from build123d import *

# Parameters (mm, degrees)
SKETCH2_R            = 13
SKETCH2_R_2          = 10
BOSS_EXTRUDE3_DEPTH  = 100
SKETCH2_3_R          = 14.5
SKETCH2_3_R_2        = 13
BOSS_EXTRUDE5_DEPTH  = 10
SKETCH8_R            = 25
BOSS_EXTRUDE7_DEPTH  = 6
SKETCH11_R           = 5.5
BOSS_EXTRUDE12_DEPTH = 10
SKETCH14_W           = 47.941155358
SKETCH14_H           = 10.12177459
CUT_EXTRUDE2_DEPTH   = 112.740771431
FILLET1_START        = -12.0000001
FILLET1_2_DEPTH      = 2.0000001
FILLET1_START_2      = 3.060887195
FILLET1_3_DEPTH      = 2.0000001
FILLET1_START_3      = -5.060887295
FILLET1_4_DEPTH      = 2
FILLET1_START_4      = 10
FILLET1_5_DEPTH      = 2
FILLET1_START_5      = -10
FILLET1_6_DEPTH      = 4.939112705
FILLET1_START_6      = 5.060887295
FILLET1_7_DEPTH      = 4.939112705
FILLET1_START_7      = -21.9089024
FILLET1_8_DEPTH      = 43.8178047


with BuildPart() as part:
    # Sketch2 → Boss-Extrude3 (new body)
    with BuildSketch(Plane(origin=(0, 0, 0), x_dir=(1, 0, 0), z_dir=(0, 1, 0))):
        with Locations(Location((0, 0, 0), (0, 0, 270))):
            Circle(SKETCH2_R)
        with Locations(Location((0, 0, 0), (0, 0, 270))):
            Circle(SKETCH2_R_2, mode=Mode.SUBTRACT)
    extrude(amount=BOSS_EXTRUDE3_DEPTH)

    # Sketch2<3> → Boss-Extrude5 (add)
    with BuildSketch(Plane(origin=(0, 0, 0), x_dir=(1, 0, 0), z_dir=(0, 1, 0))):
        with Locations(Location((0, 0, 0), (0, 0, 270))):
            Circle(SKETCH2_3_R)
        with Locations(Location((0, 0, 0), (0, 0, 270))):
            Circle(SKETCH2_3_R_2, mode=Mode.SUBTRACT)
    extrude(amount=BOSS_EXTRUDE5_DEPTH)

    # Sketch8 → Boss-Extrude7 (add)
    with BuildSketch(Plane(origin=(0, 100, 0), x_dir=(1, 0, 0), z_dir=(0, 1, 0))):
        with Locations(Location((0, 0, 0), (0, 0, 270))):
            Circle(SKETCH8_R)
    extrude(amount=BOSS_EXTRUDE7_DEPTH)

    # Sketch11 → Boss-Extrude12 (add, symmetric)
    with BuildSketch(Plane.XY):
        with BuildLine():
            Line((20, 106), (-20, 106))
            ThreePointArc((-20, 106), (0, 126), (20, 106))
        make_face()
        with Locations((0, 116)):
            Circle(SKETCH11_R, mode=Mode.SUBTRACT)
    extrude(amount=BOSS_EXTRUDE12_DEPTH, both=True)

    # Sketch14 → Cut-Extrude2 (cut, through all)
    with BuildSketch(Plane(origin=(0, 106, 0), x_dir=(1, 0, 0), z_dir=(0, 1, 0))):
        Rectangle(SKETCH14_W, SKETCH14_H)
    extrude(amount=CUT_EXTRUDE2_DEPTH, mode=Mode.SUBTRACT)

    # Fillet1: read off the stored shape, not the designer's step
    # Fillet1 outline → Fillet1 (revolve)
    with BuildSketch(Plane.XY):
        with BuildLine():
            Line((15, 100), (13, 100))
            Line((13, 100), (13, 98))
            ThreePointArc((13, 98), (13.585786438, 99.414213562), (15, 100))
        make_face()
        with BuildLine():
            ThreePointArc((14.5, 10), (13.41886117, 10.711746802), (13, 11.936491673))
            Line((13, 11.936491673), (13, 10))
            Line((13, 10), (14.5, 10))
        make_face()
    revolve(axis=Axis((0, 0, 0), (0, 1, 0)))

    # Fillet1 2 outline → Fillet1 2 (add)
    with BuildSketch(Plane.XY.offset(FILLET1_START)):
        with BuildLine():
            ThreePointArc((21.9089023, 106), (20.560502575, 106.522902108), (19.917183909, 107.818181818))
            ThreePointArc((19.917183909, 107.818181818), (0, 126), (-19.917183909, 107.818181818))
            ThreePointArc((-19.917183909, 107.818181818), (-20.560502575, 106.522902108), (-21.9089023, 106))
            Line((-21.9089023, 106), (21.9089023, 106))
        make_face()
    extrude(amount=FILLET1_2_DEPTH)

    # Fillet1 3 outline → Fillet1 3 (add)
    with BuildSketch(Plane.XY.offset(FILLET1_START_2)):
        with BuildLine():
            ThreePointArc((21.9089023, 106), (20.560502575, 106.522902108), (19.917183909, 107.818181818))
            ThreePointArc((19.917183909, 107.818181818), (0, 126), (-19.917183909, 107.818181818))
            ThreePointArc((-19.917183909, 107.818181818), (-20.560502575, 106.522902108), (-21.9089023, 106))
            Line((-21.9089023, 106), (21.9089023, 106))
        make_face()
    extrude(amount=FILLET1_3_DEPTH)

    # Fillet1 4 outline → Fillet1 4 (add)
    with BuildSketch(Plane.XY.offset(FILLET1_START_3)):
        with BuildLine():
            ThreePointArc((21.9089023, 106), (20.560502575, 106.522902108), (19.917183909, 107.818181818))
            ThreePointArc((19.917183909, 107.818181818), (0, 126), (-19.917183909, 107.818181818))
            ThreePointArc((-19.917183909, 107.818181818), (-20.560502575, 106.522902108), (-21.9089023, 106))
            Line((-21.9089023, 106), (21.9089023, 106))
        make_face()
    extrude(amount=FILLET1_4_DEPTH)

    # Fillet1 5 outline → Fillet1 5 (add)
    with BuildSketch(Plane.XY.offset(FILLET1_START_4)):
        with BuildLine():
            ThreePointArc((21.9089023, 106), (20.560502575, 106.522902108), (19.917183909, 107.818181818))
            ThreePointArc((19.917183909, 107.818181818), (0, 126), (-19.917183909, 107.818181818))
            ThreePointArc((-19.917183909, 107.818181818), (-20.560502575, 106.522902108), (-21.9089023, 106))
            Line((-21.9089023, 106), (21.9089023, 106))
        make_face()
    extrude(amount=FILLET1_5_DEPTH)

    # Fillet1 6 outline → Fillet1 6 (add)
    with BuildSketch(Plane.XY.offset(FILLET1_START_5)):
        with BuildLine():
            Line((20, 106), (21.9089023, 106))
            ThreePointArc((21.9089023, 106), (20.560502575, 106.522902108), (19.917183909, 107.818181818))
            ThreePointArc((19.917183909, 107.818181818), (19.97928525, 106.910033465), (20, 106))
        make_face()
        with BuildLine():
            ThreePointArc((-20, 106), (-19.97928525, 106.910033465), (-19.917183909, 107.818181818))
            ThreePointArc((-19.917183909, 107.818181818), (-20.560502575, 106.522902108), (-21.9089023, 106))
            Line((-21.9089023, 106), (-20, 106))
        make_face()
    extrude(amount=FILLET1_6_DEPTH)

    # Fillet1 7 outline → Fillet1 7 (add)
    with BuildSketch(Plane.XY.offset(FILLET1_START_6)):
        with BuildLine():
            Line((20, 106), (21.9089023, 106))
            ThreePointArc((21.9089023, 106), (20.560502575, 106.522902108), (19.917183909, 107.818181818))
            ThreePointArc((19.917183909, 107.818181818), (19.97928525, 106.910033465), (20, 106))
        make_face()
        with BuildLine():
            ThreePointArc((-20, 106), (-19.97928525, 106.910033465), (-19.917183909, 107.818181818))
            ThreePointArc((-19.917183909, 107.818181818), (-20.560502575, 106.522902108), (-21.9089023, 106))
            Line((-21.9089023, 106), (-20, 106))
        make_face()
    extrude(amount=FILLET1_7_DEPTH)

    # Fillet1 8 outline → Fillet1 8 (cut)
    with BuildSketch(Plane.YZ.offset(FILLET1_START_7)):
        with BuildLine():
            Line((108, 10), (127, 10))
            Line((127, 10), (127, 12))
            Line((127, 12), (106, 12))
            ThreePointArc((106, 12), (106.585786438, 10.585786438), (108, 10))
        make_face()
        with BuildLine():
            Line((127, 3.060887195), (127, 5.060887295))
            Line((127, 5.060887295), (108, 5.060887295))
            ThreePointArc((108, 5.060887295), (106.585786438, 4.475100858), (106, 3.060887295))
            Line((106, 3.060887295), (127, 3.060887195))
        make_face()
        with BuildLine():
            Line((127, -5.060887295), (127, -3.060887295))
            Line((127, -3.060887295), (106, -3.060887295))
            ThreePointArc((106, -3.060887295), (106.585786438, -4.475100858), (108, -5.060887295))
            Line((108, -5.060887295), (127, -5.060887295))
        make_face()
        with BuildLine():
            Line((127, -12.0000001), (127, -10))
            Line((127, -10), (108, -10))
            ThreePointArc((108, -10), (106.585786438, -10.585786438), (106, -12))
            Line((106, -12), (127, -12.0000001))
        make_face()
    extrude(amount=FILLET1_8_DEPTH, mode=Mode.SUBTRACT)


solid = part.part
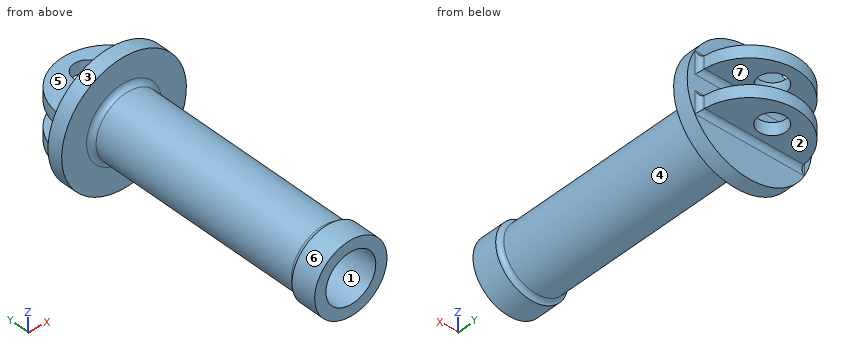
Here's how the part is built. I have some questions about the finished solid (model axes, mm). Face numbers are marked on the shaded views. A direction names the side the tool comes from. Coordinates: 2 decimals unless noted, no trailing zeros. Order: outer loops, then holes, each group sorted by start corner. A loop starts at its lowest first (then second) coordinate and runs counter-clockwise, first axis right, second up. Notation, with made-up numbers: (62.5, 77) -> (87.5, 77) arc R17 cw to (87.5, 97) -> close; hole circle Ø9 at (50.5, -24). An arc over 180 degrees is marked (long way). Answer in a Markdown table with one row per item.
(1) I want a section at B-B on y = 116. List the corners of the cut face in (x, z) for me, then the cut area to 3 significant figures.
Answer key:
| item | result |
|---|---|
| outline | (-17.32, -10) -> (-5.5, -10) -> (-5.5, -5.06) -> (-17.32, -5.06) -> close; (-17.32, 5.06) -> (-5.5, 5.06) -> (-5.5, 10) -> (-17.32, 10) -> close; (5.5, -10) -> (17.32, -10) -> (17.32, -5.06) -> (5.5, -5.06) -> close; (5.5, 5.06) -> (17.32, 5.06) -> (17.32, 10) -> (5.5, 10) -> close |
| area | 234 mm^2 |
(2) Thinking about a two-plate mould opening in Z: for the marked faces 5, 6 and 7, which applies, +Z half, -Z half, draft (parallel to the pull), parting line (faces both ways), or undercut?
Answer key:
| item | result |
|---|---|
| face 5 | +Z half |
| face 6 | parting line |
| face 7 | undercut |
(3) Please list where these lines run through material, in increasing order: probe 1 along Y at (x, z) = (0, -6.15); probe 2 along X at (y, z) = (29, 0); probe 3 along Z at (x, y) = (-6.5, 114.5).
Answer key:
| item | result |
|---|---|
| probe 1 | 100 to 110.5, 121.5 to 126 |
| probe 2 | -13 to -10, 10 to 13 |
| probe 3 | -10 to -5.06, 5.06 to 10 |
(4) I want a section at D-D on y = 64.5. List the corners of the cut face in (x, z) for me.
Answer key:
| item | result |
|---|---|
| outline | circle Ø26 at (0, 0); hole circle Ø20 at (0, 0) |
(5) I want a section at C-C on x = -16.5. List the corners of the cut face in (y, z) for me, then the cut area to 3 significant figures.
Answer key:
| item | result |
|---|---|
| outline | (100, -18.78) -> (106, -18.78) -> (106, -12) arc R2 cw to (108, -10) -> (117.3, -10) -> (117.3, -5.06) -> (108, -5.06) arc R2 cw to (106, -3.06) -> (106, 3.06) arc R2 cw to (108, 5.06) -> (117.3, 5.06) -> (117.3, 10) -> (108, 10) arc R2 cw to (106, 12) -> (106, 18.78) -> (100, 18.78) -> close |
| area | 340 mm^2 |
(6) Will these pins go through, and if not, where does the flat tip stop? pin 1 Ø12.5 at (x, y) = (0, 116) entering from +Z; pin 2 Ø20 at (x, y) = (-9, 116.5) entering from +Z; pin 3 Ø3 at (x, z) = (2, -7) entering from +Y.
Answer key:
| item | result |
|---|---|
| pin 1 | z = 10 |
| pin 2 | z = 10.68 |
| pin 3 | y = 125.99 |
(7) On a 3-axis mill with a long thin cutter (end or side, diameter ignored), from which of +Z, -Z, +X, -X, +Y, -Y can I reach the whole of each face in a straight line? I mean the marked faces 1, 2, 3 and 4. Say none if no direction works.
Answer key:
| item | result |
|---|---|
| face 1 | -Y |
| face 2 | -Z, +X, -X, +Y |
| face 3 | +Y, -Y |
| face 4 | none |
(8) I want a section at A-A on z = 0. List the corners of the cut face in (x, y) for me, then the cut area to 3 significant figures.
Answer key:
| item | result |
|---|---|
| outline | (-25, 100) -> (-15, 100) arc R2 cw to (-13, 98) -> (-13, 11.94) arc R2 cw to (-14.5, 10) -> (-14.5, 0) -> (-10, 0) -> (-10, 100) -> (10, 100) -> (10, 0) -> (14.5, 0) -> (14.5, 10) arc R2 cw to (13, 11.94) -> (13, 98) arc R2 cw to (15, 100) -> (25, 100) -> (25, 106) -> (-25, 106) -> close |
| area | 933 mm^2 |
